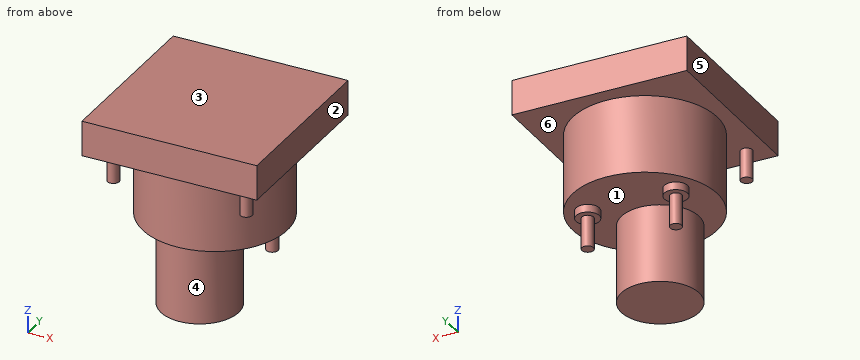
```python
from build123d import *

# Parameters (mm, degrees)
SKETCH_1_W      = 45
SKETCH_1_H      = 45
EXTRUDE_1_DEPTH = 9
SKETCH_2_R      = 18.6
EXTRUDE_2_DEPTH = 20
SKETCH_3_R      = 3
EXTRUDE_3_DEPTH = 2
SKETCH_4_R      = 1.5
EXTRUDE_4_DEPTH = 8
SKETCH_5_R      = 10
EXTRUDE_5_DEPTH = 20
SKETCH_6_R      = 1.5
EXTRUDE_6_DEPTH = 7.6


with BuildPart() as part:
    # 草图1 → 凸台-拉伸1 (new body)
    with BuildSketch(Plane.XY):
        with Locations((22.5, 22.5)):
            Rectangle(SKETCH_1_W, SKETCH_1_H)
    extrude(amount=-EXTRUDE_1_DEPTH)

    # 草图2 → 凸台-拉伸2 (add)
    with BuildSketch(Plane(origin=(0, 0, -9), x_dir=(-1, 0, 0), z_dir=(0, 0, -1))):
        with Locations((-22.5, 22.5)):
            Circle(SKETCH_2_R)
    extrude(amount=EXTRUDE_2_DEPTH)

    # 草图3 → 凸台-拉伸3 (add)
    with BuildSketch(Plane(origin=(0, 0, -29), x_dir=(-1, 0, 0), z_dir=(0, 0, -1))):
        with Locations((-33.85, 29)):
            Circle(SKETCH_3_R)
        with Locations((-11.15, 29)):
            Circle(SKETCH_3_R)
    extrude(amount=EXTRUDE_3_DEPTH)

    # 草图4 → 凸台-拉伸4 (add)
    with BuildSketch(Plane(origin=(0, 0, -31), x_dir=(-1, 0, 0), z_dir=(0, 0, -1))):
        with Locations((-33.85, 29)):
            Circle(SKETCH_4_R)
        with Locations((-11.15, 29)):
            Circle(SKETCH_4_R)
    extrude(amount=EXTRUDE_4_DEPTH)

    # 草图5 → 凸台-拉伸5 (add)
    with BuildSketch(Plane(origin=(0, 0, -29), x_dir=(-1, 0, 0), z_dir=(0, 0, -1))):
        with Locations((-22.5, 15)):
            Circle(SKETCH_5_R)
    extrude(amount=EXTRUDE_5_DEPTH)

    # 草图6 → 凸台-拉伸6 (add)
    with BuildSketch(Plane(origin=(0, 0, -9), x_dir=(-1, 0, 0), z_dir=(0, 0, -1))):
        with Locations(Location((-39.6, 5.18, 0), (0, 0, 180))):
            Circle(SKETCH_6_R)
        with Locations(Location((-5.4, 5.18, 0), (0, 0, 180))):
            Circle(SKETCH_6_R)
    extrude(amount=EXTRUDE_6_DEPTH)


solid = part.part
```
Work out the finished part from the listing and answer in its coordinate system (mm). Face numbers are marked on the shaded views. A direction names the side the tool comes from. Give positions to 0.01 mm unless a question says otherwise; leave off trailing zeros. Write each loop counter-clockwise with the first axis right and the second up, starting at its lowest first coordinate (ties: lowest second). Pieces come first, ordered by that corner, then holes. Notation, with made-up numbers: (6.25, 10) - (37.25, 10) arc R25 ccw to (37.25, 27) - close; hole circle Ø10 at (-37, 79.5). An arc over 180 degrees is marked (long way). Use one line per item in the form item = value.
1. Consider L1, parallel to Z at x = 21, y = 31.5; L2, parallel to Z at x = 9, y = 29; L3, parallel to X at y = 30, z = -33. Determine where each line is inside the solid, lowest interval first.
Filled in:
L1 = -29 to 0
L2 = -31 to 0
L3 = 10.03 to 12.27, 32.73 to 34.97
2. A cutting plane is placed at A-A (z = -12). Write down the section's boundary in (x, y).
Filled in:
outline = circle Ø3 at (5.4, 5.18); circle Ø37.2 at (22.5, 22.5); circle Ø3 at (39.6, 5.18)
3. A cutting plane is placed at B-B (x = 22.5). Write down the section's boundary in (y, z), and give its area (3 significant figures).
Filled in:
outline = (0, -9) - (3.9, -9) - (3.9, -29) - (5, -29) - (5, -49) - (25, -49) - (25, -29) - (41.1, -29) - (41.1, -9) - (45, -9) - (45, 0) - (0, 0) - close
area = 1,550 mm^2
4. A cutting plane is placed at C-C (y = 15). Write down the section's boundary in (x, z).
Filled in:
outline = (0, -9) - (5.48, -9) - (5.48, -29) - (12.5, -29) - (12.5, -49) - (32.5, -49) - (32.5, -29) - (39.52, -29) - (39.52, -9) - (45, -9) - (45, 0) - (0, 0) - close
5. Each of these flat-tipped pins is pushed along its axis until it touches: pin 1 Ø1.5 at (x, z) = (23, -39.5) entering from -Y; pin 2 Ø5 at (x, z) = (21.5, -14.5) entering from +Y; pin 3 Ø3.5 at (x, y) = (33.5, 29) entering from -Z. Where does it stop, or does it pass through?
Filled in:
pin_1 = 5
pin_2 = 41.1
pin_3 = -39
6. A cutting plane is placed at D-D (z = -37.5). Write down the section's boundary in (x, y), and give its area (3 significant figures).
Filled in:
outline = circle Ø3 at (11.15, 29); circle Ø20 at (22.5, 15); circle Ø3 at (33.85, 29)
area = 328 mm^2
7. Determine the mould class of the marked faces 1, 2, 3 and 4 for opening direction X: released by +X, released by -X, zero draft, split by the parting line, or undercut.
Filled in:
face_1 = undercut
face_2 = released by +X
face_3 = zero draft
face_4 = split by the parting line
8. For the marked faces 5 and 6, determine the directions among +Z, -Z, +X, -X, +Y, -Y from which every point of the face is accessible in a straight line to the end or side of a thin tool.
Filled in:
face_5 = +Z, -Z, -X, +Y, -Y
face_6 = -Z
